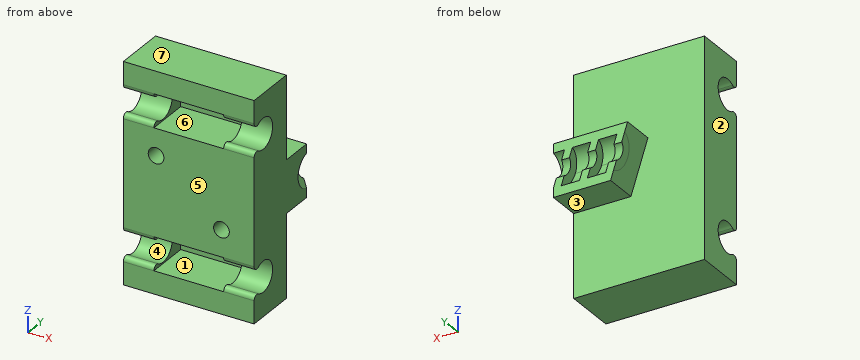
```python
from build123d import *

# Parameters (mm, degrees)
SKETCH_1_W          = 15
SKETCH_1_H          = 25
EXTRUDE_1_DEPTH     = 6
SKETCH_3_R          = 1.75
CUT_EXTRUDE_1_DEPTH = 15
FILLET_1_R          = 0.5
SKETCH_4_W          = 15
SKETCH_4_H          = 6
EXTRUDE_3_DEPTH     = 2.2
EXTRUDE_4_DEPTH     = 15
EXTRUDE_5_REACH     = 32.758
CUT_EXTRUDE_2_REACH = 32.758
SKETCH_8_R          = 1
CUT_EXTRUDE_START   = 6
CUT_EXTRUDE_3_DEPTH = 3.8
SKETCH_10_W         = 8
SKETCH_10_H         = 3.806573262
CUT_EXTRUDE_5_DEPTH = 5
SKETCH_12_R         = 0.9
CUT_EXTRUDE_7_DEPTH = 4


# Read off the part's stored shape, not the designer's step: 切除-拉伸3
with BuildPart() as part:
    # 草图1 → 凸台-拉伸1 (new body)
    with BuildSketch(Plane(origin=(0, 0, 0), x_dir=(1, 0, 0), z_dir=(0, 1, 0))):
        with Locations((7.5, -12.5)):
            Rectangle(SKETCH_1_W, SKETCH_1_H)
    extrude(amount=EXTRUDE_1_DEPTH)

    # 草图3 → 切除-拉伸1 (cut)
    with BuildSketch(Plane(origin=(15, 0, 0), x_dir=(0, 0, -1), z_dir=(1, 0, 0))):
        with Locations((-20.5, 1.7)):
            Circle(SKETCH_3_R)
        with Locations((-4.5, 1.7)):
            Circle(SKETCH_3_R)
    extrude(amount=-CUT_EXTRUDE_1_DEPTH, mode=Mode.SUBTRACT)

    # 圆角1
    fillet_1_edges = [part.edges().sort_by_distance(p)[0] for p in [
        (7.5, 0, 4.084668807),
        (7.5, 0, 4.915331193),
        (7.5, 0, 20.084668807),
        (7.5, 0, 20.915331193),
    ]]
    fillet(fillet_1_edges, radius=FILLET_1_R)

    # 草图4 → 凸台-拉伸3 (add)
    with BuildSketch(Plane(origin=(0, 6, 0), x_dir=(1, 0, 0), z_dir=(0, 1, 0))):
        with Locations((7.5, -12.5)):
            Rectangle(SKETCH_4_W, SKETCH_4_H)
    extrude(amount=EXTRUDE_3_DEPTH)

    # 草图6 → 凸台-拉伸4 (add)
    with BuildSketch(Plane(origin=(15, 0, 0), x_dir=(0, 0, -1), z_dir=(1, 0, 0))):
        with BuildLine():
            ThreePointArc((-10.540408206, 9.8), (-11.235088936, 8.650806662), (-12.5, 8.2))
            Line((-12.5, 8.2), (-9.5, 8.2))
            Line((-9.5, 8.2), (-9.5, 9.8))
            Line((-9.5, 9.8), (-10.540408206, 9.8))
        make_face()
        with BuildLine():
            Line((-15.5, 9.8), (-15.5, 8.2))
            Line((-15.5, 8.2), (-12.5, 8.2))
            ThreePointArc((-12.5, 8.2), (-13.764911064, 8.650806662), (-14.459591794, 9.8))
            Line((-14.459591794, 9.8), (-15.5, 9.8))
        make_face()
    extrude(amount=-EXTRUDE_4_DEPTH)

    # 草图7 → 凸台-拉伸5 (add, up to next)
    with BuildSketch(Plane(origin=(0, 9.8, 0), x_dir=(1, 0, 0), z_dir=(0, 1, 0)), mode=Mode.PRIVATE) as extrude_5_sk1:
        Polygon((14.1, -10.540408206), (15, -10.540408206), (13.726580059, -14.459591794), (12.826580059, -14.459591794), align=None)
    extrude_5_tool1 = extrude(extrude_5_sk1.sketch, amount=-EXTRUDE_5_REACH, mode=Mode.PRIVATE) - part.part
    # 草图7 → 凸台-拉伸5 (add, up to next)
    with BuildSketch(Plane(origin=(0, 9.8, 0), x_dir=(1, 0, 0), z_dir=(0, 1, 0)), mode=Mode.PRIVATE) as extrude_5_sk2:
        Polygon((11.1, -10.540408206), (12, -10.540408206), (10.726580059, -14.459591794), (9.826580059, -14.459591794), align=None)
    extrude_5_tool2 = extrude(extrude_5_sk2.sketch, amount=-EXTRUDE_5_REACH, mode=Mode.PRIVATE) - part.part
    # 草图7 → 凸台-拉伸5 (add, up to next)
    with BuildSketch(Plane(origin=(0, 9.8, 0), x_dir=(1, 0, 0), z_dir=(0, 1, 0)), mode=Mode.PRIVATE) as extrude_5_sk3:
        Polygon((8.1, -10.540408206), (9, -10.540408206), (7.726580059, -14.459591794), (6.826580059, -14.459591794), align=None)
    extrude_5_tool3 = extrude(extrude_5_sk3.sketch, amount=-EXTRUDE_5_REACH, mode=Mode.PRIVATE) - part.part
    # 草图7 → 凸台-拉伸5 (add, up to next)
    with BuildSketch(Plane(origin=(0, 9.8, 0), x_dir=(1, 0, 0), z_dir=(0, 1, 0)), mode=Mode.PRIVATE) as extrude_5_sk4:
        Polygon((5.1, -10.540408206), (6, -10.540408206), (4.726580059, -14.459591794), (3.826580059, -14.459591794), align=None)
    extrude_5_tool4 = extrude(extrude_5_sk4.sketch, amount=-EXTRUDE_5_REACH, mode=Mode.PRIVATE) - part.part
    # 草图7 → 凸台-拉伸5 (add, up to next)
    with BuildSketch(Plane(origin=(0, 9.8, 0), x_dir=(1, 0, 0), z_dir=(0, 1, 0)), mode=Mode.PRIVATE) as extrude_5_sk5:
        Polygon((2.1, -10.540408206), (3, -10.540408206), (1.726580059, -14.459591794), (0.826580059, -14.459591794), align=None)
    extrude_5_tool5 = extrude(extrude_5_sk5.sketch, amount=-EXTRUDE_5_REACH, mode=Mode.PRIVATE) - part.part
    add(extrude_5_tool1.solids().sort_by_distance((13.91329, 9.8, 12.5))[0])
    add(extrude_5_tool2.solids().sort_by_distance((10.91329, 9.8, 12.5))[0])
    add(extrude_5_tool3.solids().sort_by_distance((7.91329, 9.8, 12.5))[0])
    add(extrude_5_tool4.solids().sort_by_distance((4.91329, 9.8, 12.5))[0])
    add(extrude_5_tool5.solids().sort_by_distance((1.91329, 9.8, 12.5))[0])

    # 切除-拉伸2: up to this face of the body (flat: up to its plane)
    cut_extrude_2_end = Plane(part.part.faces().sort_by_distance((0, 3.752278375, 12.5))[0])
    # 草图8 → 切除-拉伸2 (cut, up to the picked face)
    with BuildSketch(Plane(origin=(15, 0, 0), x_dir=(0, 0, -1), z_dir=(1, 0, 0)), mode=Mode.PRIVATE) as cut_extrude_2_sk1:
        with Locations((-12.5, 10.2)):
            Circle(SKETCH_8_R)
    cut_extrude_2_tool1 = split(extrude(cut_extrude_2_sk1.sketch, amount=-CUT_EXTRUDE_2_REACH, mode=Mode.PRIVATE), bisect_by=cut_extrude_2_end, keep=Keep.BOTH, mode=Mode.PRIVATE)
    add(cut_extrude_2_tool1.solids().sort_by(Axis((15, 10.2, 12.5), (-1, 0, 0)))[0], mode=Mode.SUBTRACT)

    # 切除-拉伸3 outline → 切除-拉伸3 (cut)
    with BuildSketch(Plane(origin=(0, 0, 0), x_dir=(1, 0, 0), z_dir=(0, 1, 0)).offset(CUT_EXTRUDE_START)):
        Polygon((6.488530941, -15.5), (8.438049118, -9.5), (0, -9.5), (0, -15.5), align=None)
    extrude(amount=CUT_EXTRUDE_3_DEPTH, mode=Mode.SUBTRACT)

    # 草图10 → 切除-拉伸5 (cut)
    with BuildSketch(Plane.XZ):
        with Locations((7.5, 20.5)):
            Rectangle(SKETCH_10_W, SKETCH_10_H)
        with Locations((7.5, 4.5)):
            Rectangle(SKETCH_10_W, SKETCH_10_H)
    extrude(amount=-CUT_EXTRUDE_5_DEPTH, mode=Mode.SUBTRACT)

    # 草图12 → 切除-拉伸7 (cut)
    with BuildSketch(Plane.XZ):
        with Locations(Location((11.25, 9.451643316, 0), (0, 0, 270))):
            Circle(SKETCH_12_R)
        with Locations(Location((3.75, 15.548356684, 0), (0, 0, 90))):
            Circle(SKETCH_12_R)
    extrude(amount=-CUT_EXTRUDE_7_DEPTH, mode=Mode.SUBTRACT)


solid = part.part
```
Read the model definition and answer for the solid it produces. Units are mm, in the model's axes. Face numbers are marked on the shaded views. A direction names the side the tool comes from. Coordinates: 2 decimals unless noted, no trailing zeros. Loops run counter-clockwise (first coordinate to the right, second up) from the corner with the lowest first, then second, coordinate; pieces in that order, holes last.
(1) The part is cut by section D-D (y = 7.25). Determine the outline of the cut face in (x, z), and give its area (3 significant figures).
Solution:
outline: (6.49, 15.5) - (8.44, 9.5) - (15, 9.5) - (15, 15.5) - close
area: 45.2 mm2
(2) The part is cut by section C-C (x = 3.75). Determine the outline of the cut face in (y, z), and give its area (3 significant figures).
Solution:
outline: (0, 0) - (6, 0) - (6, 25) - (0, 25) - (0, 22.4) - (5, 22.4) - (5, 18.6) - (0, 18.6) - (0, 16.45) - (4, 16.45) - (4, 14.65) - (0, 14.65) - (0, 6.4) - (5, 6.4) - (5, 2.6) - (0, 2.6) - close
area: 105 mm2
(3) The part is cut by section B-B (z = 4.5). Determine the outline of the cut face in (x, y), and give its area (4 significant figures).
Solution:
outline: (0, 3.45) - (3.5, 3.45) - (3.5, 5) - (11.5, 5) - (11.5, 3.45) - (15, 3.45) - (15, 6) - (0, 6) - close
area: 25.85 mm2
(4) A tool of negligible diameter and unlimited length cuts with its end or side. For the marked faces 1, 2 and 3, from which of +Z, -Z, +X, -X, +Y, -Y can it reach the whole face along a straight path? Write none if from no direction.
Solution:
face 1: -Y
face 2: +Z, -Z, -X, +Y, -Y
face 3: -Z, +X, -X, +Y
(5) The part is cut by section A-A (y = 2.75). Count the separate pieces of the cut face and the enclosed holes in it, and give its area (3 significant figures).
Solution:
separate pieces: 3
enclosed holes: 2
area: 270 mm2
(6) Flat-ended cylindrical pins translate along their axes: pin 1 Ø1 at (x, z) = (5, 17) entering from +Y; pin 2 Ø1.9 at (x, z) = (7.5, 4) entering from -Y. Find the tip coordinate at first contact, or state that the pin passes through.
Solution:
pin 1: stops at y = 6
pin 2: stops at y = 5
(7) Consider line 1 along Z through (x, y) = (12.35, 1.7); line 2 along Z through (x, y) = (7.25, 2); line 3 along Z through (x, y) = (11, 1). Determine where each line is inside the solid, lowest interval first.
Solution:
line 1: z = 0 to 2.75, 6.25 to 18.75, 22.25 to 25
line 2: z = 0 to 2.6, 6.4 to 18.6, 22.4 to 25
line 3: z = 0 to 2.6, 6.4 to 8.59, 10.32 to 18.6, 22.4 to 25
(8) The mould has two halves that part along Z. Classify the marked faces 4, 5, 6 and 7: released by +Z, released by -Z, zero draft, split by the parting line, or undercut.
Solution:
face 4: undercut
face 5: zero draft
face 6: undercut
face 7: released by +Z
